```python
from build123d import *

# Parameters (mm, degrees)
SKETCH1_W           = 400
SKETCH1_H           = 100
BOSS_EXTRUDE1_DEPTH = 3
SKETCH2_R           = 2.5
SKETCH2_R_2         = 39
CUT_EXTRUDE1_DEPTH  = 207.177108332
CUT_EXTRUDE2_DEPTH  = 207.177108332
CUT_EXTRUDE3_REACH  = 208.177
SKETCH4_R           = 2.5
SKETCH5_R           = 2.5
CUT_EXTRUDE4_DEPTH  = 207.177108332
CUT_EXTRUDE5_REACH  = 208.177
SKETCH6_W           = 21
SKETCH6_H           = 7


with BuildPart() as part:
    # Sketch1 → Boss-Extrude1 (new body)
    with BuildSketch(Plane.XY):
        Rectangle(SKETCH1_W, SKETCH1_H)
    extrude(amount=BOSS_EXTRUDE1_DEPTH)

    # Sketch2 → Cut-Extrude1 (cut, through all)
    with BuildSketch(Plane.XY.offset(3)):
        with Locations((-64.25, 35.75)):
            Circle(SKETCH2_R)
        with Locations((-64.25, -35.75)):
            Circle(SKETCH2_R)
        with Locations((-135.75, -35.75)):
            Circle(SKETCH2_R)
        with Locations((-135.75, 35.75)):
            Circle(SKETCH2_R)
        with Locations((-100, 0)):
            Circle(SKETCH2_R_2)
        with Locations(Location((100, 0, 0), (0, 0, 180))):
            Circle(SKETCH2_R_2)
        with Locations(Location((135.75, 35.75, 0), (0, 0, 180))):
            Circle(SKETCH2_R)
        with Locations(Location((135.75, -35.75, 0), (0, 0, 180))):
            Circle(SKETCH2_R)
        with Locations(Location((64.25, -35.75, 0), (0, 0, 180))):
            Circle(SKETCH2_R)
        with Locations(Location((64.25, 35.75, 0), (0, 0, 180))):
            Circle(SKETCH2_R)
    extrude(amount=-CUT_EXTRUDE1_DEPTH, mode=Mode.SUBTRACT)

    # Sketch3 → Cut-Extrude2 (cut, through all)
    with BuildSketch(Plane.XY.offset(3)):
        with BuildLine():
            Line((-50, 5), (50, 5))
            ThreePointArc((50, 5), (55, 0), (50, -5))
            Line((50, -5), (-50, -5))
            ThreePointArc((-50, -5), (-55, 0), (-50, 5))
        make_face()
        with BuildLine():
            Line((-50, 25), (50, 25))
            ThreePointArc((50, 25), (55, 20), (50, 15))
            Line((50, 15), (-50, 15))
            ThreePointArc((-50, 15), (-55, 20), (-50, 25))
        make_face()
        with BuildLine():
            Line((-50, 45), (50, 45))
            ThreePointArc((50, 45), (55, 40), (50, 35))
            Line((50, 35), (-50, 35))
            ThreePointArc((-50, 35), (-55, 40), (-50, 45))
        make_face()
        with BuildLine():
            Line((-50, -45), (50, -45))
            ThreePointArc((50, -45), (55, -40), (50, -35))
            Line((50, -35), (-50, -35))
            ThreePointArc((-50, -35), (-55, -40), (-50, -45))
        make_face()
        with BuildLine():
            Line((-50, -25), (50, -25))
            ThreePointArc((50, -25), (55, -20), (50, -15))
            Line((50, -15), (-50, -15))
            ThreePointArc((-50, -15), (-55, -20), (-50, -25))
        make_face()
    extrude(amount=-CUT_EXTRUDE2_DEPTH, mode=Mode.SUBTRACT)

    # Sketch4 → Cut-Extrude3 (cut, up to next)
    with BuildSketch(Plane.XY.offset(3), mode=Mode.PRIVATE) as cut_extrude3_sk1:
        with Locations((-155, -30.5)):
            Circle(SKETCH4_R)
    cut_extrude3_tool1 = extrude(cut_extrude3_sk1.sketch, amount=-CUT_EXTRUDE3_REACH, mode=Mode.PRIVATE) & part.part
    # Sketch4 → Cut-Extrude3 (cut, up to next)
    with BuildSketch(Plane.XY.offset(3), mode=Mode.PRIVATE) as cut_extrude3_sk2:
        with Locations((-155, 30.5)):
            Circle(SKETCH4_R)
    cut_extrude3_tool2 = extrude(cut_extrude3_sk2.sketch, amount=-CUT_EXTRUDE3_REACH, mode=Mode.PRIVATE) & part.part
    # Sketch4 → Cut-Extrude3 (cut, up to next)
    with BuildSketch(Plane.XY.offset(3), mode=Mode.PRIVATE) as cut_extrude3_sk3:
        with Locations((155, 30.5)):
            Circle(SKETCH4_R)
    cut_extrude3_tool3 = extrude(cut_extrude3_sk3.sketch, amount=-CUT_EXTRUDE3_REACH, mode=Mode.PRIVATE) & part.part
    # Sketch4 → Cut-Extrude3 (cut, up to next)
    with BuildSketch(Plane.XY.offset(3), mode=Mode.PRIVATE) as cut_extrude3_sk4:
        with Locations((155, -30.5)):
            Circle(SKETCH4_R)
    cut_extrude3_tool4 = extrude(cut_extrude3_sk4.sketch, amount=-CUT_EXTRUDE3_REACH, mode=Mode.PRIVATE) & part.part
    add(cut_extrude3_tool1.solids().sort_by_distance((-155, -30.5, 3))[0], mode=Mode.SUBTRACT)
    add(cut_extrude3_tool2.solids().sort_by_distance((-155, 30.5, 3))[0], mode=Mode.SUBTRACT)
    add(cut_extrude3_tool3.solids().sort_by_distance((155, 30.5, 3))[0], mode=Mode.SUBTRACT)
    add(cut_extrude3_tool4.solids().sort_by_distance((155, -30.5, 3))[0], mode=Mode.SUBTRACT)

    # Sketch5 → Cut-Extrude4 (cut, through all)
    with BuildSketch(Plane.XY.offset(3)):
        with Locations((-180.5, -40)):
            Circle(SKETCH5_R)
        with Locations((-180.5, 40)):
            Circle(SKETCH5_R)
        with Locations(Location((180.5, 40, 0), (0, 0, 180))):
            Circle(SKETCH5_R)
        with Locations(Location((180.5, -40, 0), (0, 0, 180))):
            Circle(SKETCH5_R)
    extrude(amount=-CUT_EXTRUDE4_DEPTH, mode=Mode.SUBTRACT)

    # Sketch6 → Cut-Extrude5 (cut, up to next)
    with BuildSketch(Plane.XY.offset(3), mode=Mode.PRIVATE) as cut_extrude5_sk1:
        with Locations((-155, 46.5)):
            Rectangle(SKETCH6_W, SKETCH6_H)
    cut_extrude5_tool1 = extrude(cut_extrude5_sk1.sketch, amount=-CUT_EXTRUDE5_REACH, mode=Mode.PRIVATE) & part.part
    # Sketch6 → Cut-Extrude5 (cut, up to next)
    with BuildSketch(Plane.XY.offset(3), mode=Mode.PRIVATE) as cut_extrude5_sk2:
        with Locations((155, 46.5)):
            Rectangle(SKETCH6_W, SKETCH6_H)
    cut_extrude5_tool2 = extrude(cut_extrude5_sk2.sketch, amount=-CUT_EXTRUDE5_REACH, mode=Mode.PRIVATE) & part.part
    add(cut_extrude5_tool1.solids().sort_by_distance((-155, 46.5, 3))[0], mode=Mode.SUBTRACT)
    add(cut_extrude5_tool2.solids().sort_by_distance((155, 46.5, 3))[0], mode=Mode.SUBTRACT)


solid = part.part
```
Part model, mm, in its own coordinate system. Round coordinates to 2 decimals unless told otherwise and drop trailing zeros. Loops run counter-clockwise (first coordinate to the right, second up) from the corner with the lowest first, then second, coordinate; pieces in that order, holes last.
1. Slice it at B-B (y = 20). Give the cut face in (x, z), and give its area (3 significant figures).
Solutions:
outline: (-200, 0) - (-133.48, 0) - (-133.48, 3) - (-200, 3) - close; (-66.52, 0) - (-55, 0) - (-55, 3) - (-66.52, 3) - close; (55, 0) - (66.52, 0) - (66.52, 3) - (55, 3) - close; (133.48, 0) - (200, 0) - (200, 3) - (133.48, 3) - close
area: 468 mm2
2. Slice it at C-C (y = 0). Give the cut face in (x, z).
Solutions:
outline: (-200, 0) - (-139, 0) - (-139, 3) - (-200, 3) - close; (-61, 0) - (-55, 0) - (-55, 3) - (-61, 3) - close; (55, 0) - (61, 0) - (61, 3) - (55, 3) - close; (139, 0) - (200, 0) - (200, 3) - (139, 3) - close
3. Two-plate mould, pull along Y, no slides. Class faces 1 (the face through (-3, 12, 3)), 2 (the face through (105.077, -38.668, 1.521)), 3 (the face through (-105.077, 38.668, 1.521)): pulls with the +Y half, pulls with the -Y half, needs draft (parallel to the pull), parting line crosses it, or undercut.
Solutions:
face 1: needs draft
face 2: undercut
face 3: undercut
4. Slice it at D-D (z = 0.55). Count the separate pieces of the cut face and the enclosed holes in it, and give its area (3 significant figures).
Solutions:
separate pieces: 1
enclosed holes: 23
area: 24,400 mm2
5. Slice it at A-A (x = -100). Give the cut face in (y, z).
Solutions:
outline: (-50, 0) - (-39, 0) - (-39, 3) - (-50, 3) - close; (39, 0) - (50, 0) - (50, 3) - (39, 3) - close
6. Drill centre lines: line 1 along Y through (x, z) = (-180.5, 1.8); line 2 along Y through (x, z) = (21, 0.3); line 3 along Y through (x, z) = (155, 2.3). Where is each one in solid material? Low to high.
Solutions:
line 1: y = -50 to -42.5, -37.5 to 37.5, 42.5 to 50
line 2: y = -50 to -45, -35 to -25, -15 to -5, 5 to 15, 25 to 35, 45 to 50
line 3: y = -50 to -33, -28 to 28, 33 to 43
